Geometry: final body of the model. Coordinates: model frame, mm. A direction names the side the tool comes from. Coordinates: 2 decimals unless noted, no trailing zeros. Write each loop counter-clockwise with the first axis right and the second up, starting at its lowest first coordinate (ties: lowest second). Pieces come first, ordered by that corner, then holes. Notation, with made-up numbers: (72.5, 25) - (102.5, 25) arc R26 cw to (102.5, 53) - close; hole circle Ø6 at (8.5, 64.5). An arc over 180 degrees is marked (long way). Answer as a JSON object with one key per item and string values. Group by question number.
Item 1: Section B-B on z = 90. State how many separate pieces and enclosed holes the cut face has, and give its area (3 significant figures).
Item 2: Line query: line 1 along Y through (x, z) = (33.5, 185.5); line 2 along X through (y, z) = (0.5, 139); line 3 along Y through (x, z) = (-20.5, 402.5). Output: solid intervals per line, ascending. Write a range as from..to.
Item 3: Set-up query: faces 1 (the flat face through (0, 17.75, 325)), 2 (the flat face through (40, -11, 325)). Return all of +Z, -Z, +X, -X, +Y, -Y with unobstructed straight access to the full face (end or side cutting, diameter ignored); none if empty.
Item 4: First-contact query: pin 1 Ø1 at (y, z) = (2, 328.5) entering from +X; pin 2 Ø1 at (x, y) = (16.5, 14) entering from +Z. Flat tips, straight axial feed; report the tip coordinate or a pass-through.
Item 5: Section A-A on x = 1.5. Return loops of the section in (y, z), and give its area (3 significant figures).
Item 6: Mould query, pull axis X, two halves, no side actions, for faces 3 (the flat face through (9.4, 9.2, 0)), 4 (the flat face through (-12.91, 0, 325)), 5 (the flat face through (-40, -12, 325)). Classes: pulls with the +X half, pulls with the -X half, needs draft (parallel to the pull), parting line crosses it, or undercut.
```python
from build123d import *

# Parameters (mm, degrees)
SZKIC1_R                    = 3.4
DODANIE_WYCI_GNI_CIE1_DEPTH = 660
SZKIC2_W                    = 2.25
SZKIC2_H                    = 8
WYTNIJ_WYCI_GNI_CIE1_DEPTH  = 662.513416342


with BuildPart() as part:
    # Szkic1 → Dodanie-wyciągnięcie1 (new body)
    with BuildSketch(Plane.XY):
        with BuildLine():
            Line((-40, -19), (-40, 19))
            ThreePointArc((-40, 19), (-39.707106781, 19.707106781), (-39, 20))
            Line((-39, 20), (-24, 20))
            Line((-24, 20), (-24, 15.5))
            Line((-24, 15.5), (-26.471381771, 15.5))
            Line((-26.471381771, 15.5), (-26.471381771, 17.75))
            ThreePointArc((-26.471381771, 17.75), (-28.062372029, 17.090990258), (-28.721381771, 15.5))
            ThreePointArc((-28.721381771, 15.5), (-27.448087912, 10.962546258), (-24, 7.75))
            Line((-24, 7.75), (-16, 7.75))
            ThreePointArc((-16, 7.75), (-12.551912088, 10.962546258), (-11.278618229, 15.5))
            ThreePointArc((-11.278618229, 15.5), (-11.937627971, 17.090990258), (-13.528618229, 17.75))
            Line((-13.528618229, 17.75), (-13.528618229, 15.5))
            Line((-13.528618229, 15.5), (-16, 15.5))
            Line((-16, 15.5), (-16, 20))
            Line((-16, 20), (13.528618229, 20))
            Line((13.528618229, 20), (16, 20))
            Line((16, 20), (16, 15.5))
            Line((16, 15.5), (13.528618229, 15.5))
            Line((13.528618229, 15.5), (13.528618229, 17.75))
            ThreePointArc((13.528618229, 17.75), (11.937627971, 17.090990258), (11.278618229, 15.5))
            ThreePointArc((11.278618229, 15.5), (12.551912088, 10.962546258), (16, 7.75))
            Line((16, 7.75), (24, 7.75))
            ThreePointArc((24, 7.75), (27.448087912, 10.962546258), (28.721381771, 15.5))
            ThreePointArc((28.721381771, 15.5), (28.062372029, 17.090990258), (26.471381771, 17.75))
            Line((26.471381771, 17.75), (26.471381771, 15.5))
            Line((26.471381771, 15.5), (24, 15.5))
            Line((24, 15.5), (24, 20))
            Line((24, 20), (39, 20))
            ThreePointArc((39, 20), (39.707106781, 19.707106781), (40, 19))
            Line((40, 19), (40, 4))
            Line((40, 4), (35.5, 4))
            Line((35.5, 4), (35.5, 6.471381771))
            Line((35.5, 6.471381771), (37.75, 6.471381771))
            ThreePointArc((37.75, 6.471381771), (37.090990258, 8.062372029), (35.5, 8.721381771))
            ThreePointArc((35.5, 8.721381771), (30.962546258, 7.448087912), (27.75, 4))
            Line((27.75, 4), (27.75, -4))
            ThreePointArc((27.75, -4), (30.962546258, -7.448087912), (35.5, -8.721381771))
            ThreePointArc((35.5, -8.721381771), (37.090990258, -8.062372029), (37.75, -6.471381771))
            Line((37.75, -6.471381771), (35.5, -6.471381771))
            Line((35.5, -6.471381771), (35.5, -4))
            Line((35.5, -4), (40, -4))
            Line((40, -4), (40, -19))
            ThreePointArc((40, -19), (39.707106781, -19.707106781), (39, -20))
            Line((39, -20), (24, -20))
            Line((24, -20), (24, -15.5))
            Line((24, -15.5), (26.471381771, -15.5))
            Line((26.471381771, -15.5), (26.471381771, -17.75))
            ThreePointArc((26.471381771, -17.75), (28.062372029, -17.090990258), (28.721381771, -15.5))
            ThreePointArc((28.721381771, -15.5), (27.448087912, -10.962546258), (24, -7.75))
            Line((24, -7.75), (16, -7.75))
            ThreePointArc((16, -7.75), (12.551912088, -10.962546258), (11.278618229, -15.5))
            ThreePointArc((11.278618229, -15.5), (11.937627971, -17.090990258), (13.528618229, -17.75))
            Line((13.528618229, -17.75), (13.528618229, -15.5))
            Line((13.528618229, -15.5), (16, -15.5))
            Line((16, -15.5), (16, -20))
            Line((16, -20), (-16, -20))
            Line((-16, -20), (-16, -15.5))
            Line((-16, -15.5), (-13.528618229, -15.5))
            Line((-13.528618229, -15.5), (-13.528618229, -17.75))
            ThreePointArc((-13.528618229, -17.75), (-11.937627971, -17.090990258), (-11.278618229, -15.5))
            ThreePointArc((-11.278618229, -15.5), (-12.551912088, -10.962546258), (-16, -7.75))
            Line((-16, -7.75), (-24, -7.75))
            ThreePointArc((-24, -7.75), (-27.448087912, -10.962546258), (-28.721381771, -15.5))
            ThreePointArc((-28.721381771, -15.5), (-28.062372029, -17.090990258), (-26.471381771, -17.75))
            Line((-26.471381771, -17.75), (-26.471381771, -15.5))
            Line((-26.471381771, -15.5), (-24, -15.5))
            Line((-24, -15.5), (-24, -20))
            Line((-24, -20), (-39, -20))
            ThreePointArc((-39, -20), (-39.707106781, -19.707106781), (-40, -19))
        make_face()
        with Locations((-20, 0)):
            Circle(SZKIC1_R, mode=Mode.SUBTRACT)
        with Locations((20, 0)):
            Circle(SZKIC1_R, mode=Mode.SUBTRACT)
        with BuildLine():
            Line((30.971381771, -17.75), (36.75, -17.75))
            ThreePointArc((36.75, -17.75), (37.457106781, -17.457106781), (37.75, -16.75))
            Line((37.75, -16.75), (37.75, -10.971381771))
            Line((37.75, -10.971381771), (30.971381771, -10.971381771))
            Line((30.971381771, -10.971381771), (30.971381771, -17.75))
        make_face(mode=Mode.SUBTRACT)
        with BuildLine():
            Line((-35.5, -6.471381771), (-37.75, -6.471381771))
            ThreePointArc((-37.75, -6.471381771), (-37.090990258, -8.062372029), (-35.5, -8.721381771))
            ThreePointArc((-35.5, -8.721381771), (-30.962546258, -7.448087912), (-27.75, -4))
            Line((-27.75, -4), (-27.75, 4))
            ThreePointArc((-27.75, 4), (-30.962546258, 7.448087912), (-35.5, 8.721381771))
            ThreePointArc((-35.5, 8.721381771), (-37.090990258, 8.062372029), (-37.75, 6.471381771))
            Line((-37.75, 6.471381771), (-35.5, 6.471381771))
            Line((-35.5, 6.471381771), (-35.5, 4))
            Line((-35.5, 4), (-37.75, 4))
            Line((-37.75, 4), (-37.75, -4))
            Line((-37.75, -4), (-35.5, -4))
            Line((-35.5, -4), (-35.5, -6.471381771))
        make_face(mode=Mode.SUBTRACT)
        with BuildLine():
            Line((10.528618229, 7.090188806), (11.40950808, 7.090188806))
            ThreePointArc((11.40950808, 7.090188806), (12.470168251, 6.650848977), (12.90950808, 5.590188806))
            Line((12.90950808, 5.590188806), (12.90950808, -5.590188806))
            ThreePointArc((12.90950808, -5.590188806), (12.470168251, -6.650848977), (11.40950808, -7.090188806))
            Line((11.40950808, -7.090188806), (10.528618229, -7.090188806))
            ThreePointArc((10.528618229, -7.090188806), (9.467958057, -7.529528634), (9.028618229, -8.590188806))
            Line((9.028618229, -8.590188806), (9.028618229, -16.25))
            ThreePointArc((9.028618229, -16.25), (8.589278401, -17.310660172), (7.528618229, -17.75))
            Line((7.528618229, -17.75), (-7.528618229, -17.75))
            ThreePointArc((-7.528618229, -17.75), (-8.589278401, -17.310660172), (-9.028618229, -16.25))
            Line((-9.028618229, -16.25), (-9.028618229, -8.590188806))
            ThreePointArc((-9.028618229, -8.590188806), (-9.467958057, -7.529528634), (-10.528618229, -7.090188806))
            Line((-10.528618229, -7.090188806), (-11.40950808, -7.090188806))
            ThreePointArc((-11.40950808, -7.090188806), (-12.470168251, -6.650848977), (-12.90950808, -5.590188806))
            Line((-12.90950808, -5.590188806), (-12.90950808, 5.590188806))
            ThreePointArc((-12.90950808, 5.590188806), (-12.470168251, 6.650848977), (-11.40950808, 7.090188806))
            Line((-11.40950808, 7.090188806), (-10.528618229, 7.090188806))
            ThreePointArc((-10.528618229, 7.090188806), (-9.467958057, 7.529528634), (-9.028618229, 8.590188806))
            Line((-9.028618229, 8.590188806), (-9.028618229, 16.25))
            ThreePointArc((-9.028618229, 16.25), (-8.589278401, 17.310660172), (-7.528618229, 17.75))
            Line((-7.528618229, 17.75), (7.528618229, 17.75))
            ThreePointArc((7.528618229, 17.75), (8.589278401, 17.310660172), (9.028618229, 16.25))
            Line((9.028618229, 16.25), (9.028618229, 8.590188806))
            ThreePointArc((9.028618229, 8.590188806), (9.467958057, 7.529528634), (10.528618229, 7.090188806))
        make_face(mode=Mode.SUBTRACT)
        with BuildLine():
            Line((30.971381771, 10.971381771), (37.75, 10.971381771))
            Line((37.75, 10.971381771), (37.75, 16.75))
            ThreePointArc((37.75, 16.75), (37.457106781, 17.457106781), (36.75, 17.75))
            Line((36.75, 17.75), (30.971381771, 17.75))
            Line((30.971381771, 17.75), (30.971381771, 10.971381771))
        make_face(mode=Mode.SUBTRACT)
        with BuildLine():
            Line((-30.971381771, -10.971381771), (-30.971381771, -17.75))
            Line((-30.971381771, -17.75), (-36.75, -17.75))
            ThreePointArc((-36.75, -17.75), (-37.457106781, -17.457106781), (-37.75, -16.75))
            Line((-37.75, -16.75), (-37.75, -10.971381771))
            Line((-37.75, -10.971381771), (-30.971381771, -10.971381771))
        make_face(mode=Mode.SUBTRACT)
        with BuildLine():
            Line((-30.971381771, 17.75), (-36.75, 17.75))
            ThreePointArc((-36.75, 17.75), (-37.457106781, 17.457106781), (-37.75, 16.75))
            Line((-37.75, 16.75), (-37.75, 10.971381771))
            Line((-37.75, 10.971381771), (-30.971381771, 10.971381771))
            Line((-30.971381771, 10.971381771), (-30.971381771, 17.75))
        make_face(mode=Mode.SUBTRACT)
    extrude(amount=DODANIE_WYCI_GNI_CIE1_DEPTH)

    # Szkic2 → Wytnij-wyciągnięcie1 (cut, through all)
    with BuildSketch(Plane.XY.offset(660)):
        with Locations((-38.875, 0)):
            Rectangle(SZKIC2_W, SZKIC2_H)
    extrude(amount=-WYTNIJ_WYCI_GNI_CIE1_DEPTH, mode=Mode.SUBTRACT)


solid = part.part
```
Checks:
{
 "1": {"separate pieces": "1", "enclosed holes": "7", "area": "1,250 mm^2"},
 "2": {"line 1": "-20..-17.75, -10.97..-8.49, 8.49..10.97, 17.75..20", "line 2": "-27.75..-23.36, -16.64..-12.91, 12.91..16.64, 23.36..27.75", "line 3": "-7.75..-3.36, 3.36..7.75"},
 "3": {"face 1": "+Z, -Z", "face 2": "+Z, -Z, +X, +Y, -Y"},
 "4": {"pin 1": "x = 27.75", "pin 2": "through"},
 "5": {"outline": "(-20, 0) - (-17.75, 0) - (-17.75, 660) - (-20, 660) - close; (17.75, 0) - (20, 0) - (20, 660) - (17.75, 660) - close", "area": "2,970 mm^2"},
 "6": {"face 3": "needs draft", "face 4": "undercut", "face 5": "pulls with the -X half"}
}
